```python
from build123d import *

# Parameters (mm, degrees)
F1_W            = 10
F1_H            = 40
F1_W_2          = 180
F2_DEPTH        = 40
F3_D            = 12.1
F4_W            = 300
F4_H            = 200
F5_DEPTH        = 40
F6_SIZE         = 10
F7_SIZE         = 10
F8_SIZE         = 10
F9_R            = 10
F10_SIZE        = 5
F12_D           = 17.5
F12_CBORE_D     = 31.5
F12_CBORE_DEPTH = 20


with BuildPart() as f2:
    # F1 (on Right) → F2 (new body)
    with BuildSketch(Plane.YZ):
        with Locations((5, 20)):
            Rectangle(F1_W, F1_H)
        with Locations((100, 20)):
            Rectangle(F1_W_2, F1_H)
        with BuildLine():
            Line((0, 200), (0, 40))
            Line((0, 40), (10, 40))
            Line((10, 40), (190, 40))
            Line((190, 40), (200, 40))
            Line((200, 40), (200, 200))
            ThreePointArc((200, 200), (100, 100), (0, 200))
        make_face()
        with Locations((195, 20)):
            Rectangle(F1_W, F1_H)
        with BuildLine():
            ThreePointArc((200, 200), (100, 300), (0, 200))
            Line((0, 200), (50, 200))
            ThreePointArc((50, 200), (100, 250), (150, 200))
            Line((150, 200), (200, 200))
        make_face()
        with BuildLine():
            Line((50, 200), (0, 200))
            ThreePointArc((0, 200), (100, 100), (200, 200))
            Line((200, 200), (150, 200))
            ThreePointArc((150, 200), (100, 150), (50, 200))
        make_face()
    extrude(amount=F2_DEPTH)

    # F3 (through all)
    with Locations(Plane(origin=(0, 0, 0), x_dir=(0, 1, 0), z_dir=(-1, 0, 0))):
        with Locations((100, -272), (100, -128), (172, -200), (28, -200)):
            Hole(F3_D / 2)

    # F4 (on Top) → F5 (join)
    with BuildSketch(Plane.XY):
        with Locations((150, 100)):
            Rectangle(F4_W, F4_H)
    extrude(amount=F5_DEPTH)

    # F6
    f6_edges = [f2.edges().sort_by_distance(p)[0] for p in [
        (300, 0, 20),
    ]]
    chamfer(f6_edges, length=F6_SIZE)

    # F7
    f7_edges = [f2.edges().sort_by_distance(p)[0] for p in [
        (300, 200, 20),
    ]]
    chamfer(f7_edges, length=F7_SIZE)

    # F8
    f8_edges = [f2.edges().sort_by_distance(p)[0] for p in [
        (0, 100, 0),
    ]]
    chamfer(f8_edges, length=F8_SIZE)

    # F9
    f9_edges = [f2.edges().sort_by_distance(p)[0] for p in [
        (40, 100, 40),
    ]]
    fillet(f9_edges, radius=F9_R)

    # F10
    f10_edges = [f2.edges().sort_by_distance(p)[0] for p in [
        (40, 150, 200),
        (0, 150, 200),
    ]]
    chamfer(f10_edges, length=F10_SIZE)

    # F12 (through all)
    with Locations(Plane.XY.offset(40)):
        with Locations((268.5, 40), (148.5, 40), (148.5, 160), (268.5, 160)):
            CounterBoreHole(F12_D / 2, F12_CBORE_D / 2, F12_CBORE_DEPTH)


solid = f2.part
```
Here's how the part is built. I have some questions about the finished solid (model axes, mm). A direction names the side the tool comes from. Give positions to 0.01 mm unless a question says otherwise; leave off trailing zeros. Order: outer loops, then holes, each group sorted by start corner. A loop starts at its lowest first (then second) coordinate and runs counter-clockwise, first axis right, second up. Notation, with made-up numbers: (34, 72) -> (77, 72) arc R23 ccw to (77, 100) -> close; hole circle Ø11 at (-11.5, 5.25). An arc over 180 degrees is marked (long way). Use CSV: the item, a comma, the result in double quotes. Start each with the question number.
Item 1: Suppose I cut it at A-A (y = 40). List the corners of the cut face in (x, z) for me.
Item 2: Suppose I cut it at C-C (z = 128). List the corners of the cut face in (x, y) for me.
Item 3: Suppose I cut it at D-D (y = 100). List the corners of the cut face in (x, z) for me, and give its area (3 significant figures).
Item 4: On a 3-axis mill with a long thin cutter (end or side, diameter ignored), from which of +Z, -Z, +X, -X, +Y, -Y can I reach the whole of each face in a straight line? I mean faces 5 (the cylindrical face through (19.72, 102.199, 299.976)), 6 (the flat face through (173, 101, 40)), 7 (the flat face through (275, 33, 20)). Say none if no direction works.
Item 5: Thinking about a two-plate mould opening in Y: for faces 1 (the cylindrical face through (263.8, 167.38, 9.86)), 2 (the flat face through (40, 121, 149)), 3 (the flat face through (295, 195, 20)), 4 (the cylindrical face through (156.97, 53.28, 30.14)), which applies, pulls with the +Y half, pulls with the -Y half, needs draft (parallel to the pull), parting line crosses it, or undercut?
Item 6: Suppose I cut it at B-B (x = 268.5). List the corners of the cut face in (y, z) for me, and give its area (3 significant figures).
Item 7: I'm going to push flat-ended pins straight in: P1, Ø19.5, axis at y = 100, z = 272, coming from the +X side; P2, Ø25, axis at x = 268.5, y = 40, coming from the +Z side; P3, Ø25, axis at x = 148, y = 45.5, coming from the +Z side. Where does each tip first touch, or does it pass through?
Item 8: If I drill on probe 1 along Y at (x, z) = (268, 30); probe 2 along Y at (x, z) = (268, 6); probe 3 along Z at (x, y) = (205, 56), over which ranges is the centre line in solid material (lowest first)? Write a range as [from, to].
Answer block:
1,outline,"(0, 10) -> (10, 0) -> (139.75, 0) -> (139.75, 20) -> (132.75, 20) -> (132.75, 40) -> (50, 40) arc R10 cw to (40, 50) -> (40, 280) -> (0, 280) -> close; (157.25, 0) -> (259.75, 0) -> (259.75, 20) -> (252.75, 20) -> (252.75, 40) -> (164.25, 40) -> (164.25, 20) -> (157.25, 20) -> close; (277.25, 0) -> (300, 0) -> (300, 40) -> (284.25, 40) -> (284.25, 20) -> (277.25, 20) -> close"
2,outline,"(0, 0) -> (40, 0) -> (40, 93.95) -> (0, 93.95) -> close; (0, 106.05) -> (40, 106.05) -> (40, 200) -> (0, 200) -> close"
3,outline,"(0, 10) -> (10, 0) -> (300, 0) -> (300, 40) -> (50, 40) arc R10 cw to (40, 50) -> (40, 121.95) -> (0, 121.95) -> close; (0, 134.05) -> (40, 134.05) -> (40, 145) -> (35, 150) -> (5, 150) -> (0, 145) -> close; (0, 255) -> (5, 250) -> (35, 250) -> (40, 255) -> (40, 265.95) -> (0, 265.95) -> close; (0, 278.05) -> (40, 278.05) -> (40, 300) -> (0, 300) -> close"
3,area,"17,400 mm^2"
4,face 5,"+Z, +X, -X"
4,face 6,"+Z, +X, +Y, -Y"
4,face 7,"+Z"
5,face 1,"undercut"
5,face 2,"needs draft"
5,face 3,"pulls with the +Y half"
5,face 4,"undercut"
6,outline,"(0, 0) -> (31.25, 0) -> (31.25, 20) -> (24.25, 20) -> (24.25, 40) -> (0, 40) -> close; (48.75, 0) -> (151.25, 0) -> (151.25, 20) -> (144.25, 20) -> (144.25, 40) -> (55.75, 40) -> (55.75, 20) -> (48.75, 20) -> close; (168.75, 0) -> (200, 0) -> (200, 40) -> (175.75, 40) -> (175.75, 20) -> (168.75, 20) -> close"
6,area,"6,040 mm^2"
7,P1,"stops at x = 40"
7,P2,"stops at z = 20"
7,P3,"stops at z = 40"
8,probe 1,"y = [0, 24.26], [55.74, 144.26], [175.74, 200]"
8,probe 2,"y = [0, 31.26], [48.74, 151.26], [168.74, 200]"
8,probe 3,"z = [0, 40]"
